Check sheet for the modelled part. Datum: model origin and axes. Units: mm. A direction names the side the tool comes from. Give positions to 0.01 mm unless a question says otherwise; leave off trailing zeros. Write each loop counter-clockwise with the first axis right and the second up, starting at its lowest first coordinate (ties: lowest second). Pieces come first, ordered by that corner, then holes. Notation, with made-up numbers: M 18.25,70 L 66.25,70 A19 ccw 66.25,95 Z; hole C 6.25,17.5 d10. An arc over 180 degrees is marked long. Write item = value, one per line. Start each with the question number.
1) Access from +Z, -Z, +X, -X, +Y, -Y to the whole of each face (thin tool, end or side, straight path). Record for faces 1 (the flat face through (-2, 9, 6)), 2 (the flat face through (-2.24, -7.32, 0)).
2) Cross-section at A-A, the plane x = 0. Record the cut outline in (y, z) (3 decimals).
3) Mould release check, pull along Y, two halves, no side actions. Record for faces 3 (the cylindrical face through (7.493, -0.33, 5.577)), 4 (the flat face through (-2, -7.4, 11)), 5 (the cylindrical face through (1.172, -8.923, 8.465)): released by +Y, released by -Y, zero draft, split by the parting line, or undercut.
4) Cross-section at C-C, the plane z = 0.5. Record the cut outline in (x, y).
5) Go/stop test with flat-tipped pins: pin 1 (2 mm diameter, centred on x = 1.5, z = 8.5, fed in from +Y); pin 2 (12 mm diameter, centred on x = 0, y = 0, fed in from -Z); pin 3 (4 mm diameter, centred on y = -3.5, z = 3.5, fed in from +X). Record where each tip stops, or that it passes through.
6) Cross-section at B-B, the plane z = 9. Record the cut outline in (x, y).
7) Scan lines: line 1 along Y through (x, z) = (0, 8.75); line 2 along X through (y, z) = (0, 2.25); line 3 along Y through (x, z) = (0, 3.75). Record each from-to range of solid material in increasing order. Write a range as [from, to].
```python
from build123d import *


with BuildPart() as f1:
    # F0 (on Front) → F1 (revolve)
    with BuildSketch(Plane.XZ):
        with BuildLine():
            Line((-10.75, 0), (-7.5, 0))
            Line((-7.5, 0), (-7.5, 11))
            Line((-7.5, 11), (-9, 11))
            Line((-9, 11), (-9, 6))
            Line((-9, 6), (-10.75, 6))
            Line((-10.75, 6), (-9.107077, 4.620931))
            ThreePointArc((-9.107077, 4.620931), (-8.758565, 3.724398), (-9.32736, 2.948702))
            Line((-9.32736, 2.948702), (-10.75, 2.285273))
            Line((-10.75, 2.285273), (-10.75, 0.665314))
            Line((-10.75, 0.665314), (-10.75, 0))
        make_face()
    revolve(axis=Axis((0, 0, 13.534962), (0, 0, 1)))


solid = f1.part
```
Reply:
q1.face_1 = +Z
q1.face_2 = -Z, +X, -X, +Y, -Y
q2.outline = M -10.75,0 L -7.5,0 L -7.5,11 L -9,11 L -9,6 L -10.75,6 L -9.107,4.621 A1 cw -9.327,2.949 L -10.75,2.285 Z; M 7.5,0 L 10.75,0 L 10.75,2.285 L 9.327,2.949 A1 cw 9.107,4.621 L 10.75,6 L 9,6 L 9,11 L 7.5,11 Z
q3.face_3 = undercut
q3.face_4 = zero draft
q3.face_5 = split by the parting line
q4.outline = C 0,0 d21.5; hole C 0,0 d15
q5.pin_1 = 8.99
q5.pin_2 = through
q5.pin_3 = 10.58
q6.outline = C 0,0 d18; hole C 0,0 d15
q7.line_1 = [-9, -7.5], [7.5, 9]
q7.line_2 = [-10.75, -7.5], [7.5, 10.75]
q7.line_3 = [-8.76, -7.5], [7.5, 8.76]
